```python
from build123d import *

# Parameters (mm, degrees)
SKETCH2_W           = 15
SKETCH2_H           = 15
BOSS_EXTRUDE1_DEPTH = 15
FILLET1_R           = 6.35


with BuildPart() as part:
    # Sketch2 → Boss-Extrude1 (new body)
    with BuildSketch(Plane.XY):
        Polygon((75, 0), (75, -200), (25, -200), (25, 0), (25, 18.884295249), (0, 62.185565438), (25, 62.185565438), (25, 64.822440103), (0, 108.123710292), (25, 108.123710292), (25, 110.760584957), (0, 154.061855146), (25, 154.061855146), (25, 156.698729811), (0, 200), (100, 200), (75, 156.698729811), (75, 154.061855146), (100, 154.061855146), (75, 110.760584957), (75, 108.123710292), (100, 108.123710292), (75, 64.822440103), (75, 62.185565438), (100, 62.185565438), (75, 18.884295249), align=None)
        with Locations((50, -170)):
            Rectangle(SKETCH2_W, SKETCH2_H, mode=Mode.SUBTRACT)
        with Locations((50, -30)):
            Rectangle(SKETCH2_W, SKETCH2_H, mode=Mode.SUBTRACT)
        with Locations((50, 175)):
            Rectangle(SKETCH2_W, SKETCH2_H, mode=Mode.SUBTRACT)
    extrude(amount=-BOSS_EXTRUDE1_DEPTH)

    # Fillet1
    fillet1_edges = [part.edges().sort_by_distance(p)[0] for p in [
        (0, 62.185565438, -7.5),
        (0, 108.123710292, -7.5),
        (0, 154.061855146, -7.5),
        (0, 200, -7.5),
        (100, 200, -7.5),
        (100, 154.061855146, -7.5),
        (100, 108.123710292, -7.5),
        (100, 62.185565438, -7.5),
    ]]
    fillet(fillet1_edges, radius=FILLET1_R)


solid = part.part
```
Here's how the part is built. I have some questions about the finished solid (model axes, mm). A direction names the side the tool comes from. Coordinates: 2 decimals unless noted, no trailing zeros. Order: outer loops, then holes, each group sorted by start corner. A loop starts at its lowest first (then second) coordinate and runs counter-clockwise, first axis right, second up.
Item 1: Thinking about a two-plate mould opening in X: for faces 1 (the face through (50, 182.5, -7)), 2 (the face through (5.453, 58.93, -7.605)), 3 (the face through (94.547, 150.806, -7.605)), which applies, pulls with the +X half, pulls with the -X half, needs draft (parallel to the pull), parting line crosses it, or undercut?
Response values:
face 1: undercut
face 2: pulls with the -X half
face 3: pulls with the +X half
Item 2: Which directions (+Z, -Z, +X, -X, +Y, -Y) give clear straight access to the entire face, cutting with the end or side of a thin tool? Please do faces 4 (the face through (15.386, 127.412, -7.395)), 5 (the face through (75, -92, -7)), 6 (the face through (82, 154.062, -7)), 7 (the face through (50, -177.5, -7)), 8 (the face through (51, 3, 0)).
Response values:
face 4: +Z, -Z, -X
face 5: +Z, -Z, +X, -Y
face 6: +Z, -Z, +X
face 7: +Z, -Z
face 8: +Z, +X, -X, +Y, -Y
Item 3: If we section it at C-C, the plane y = -96: List the corners of the cut face in (x, z) for me, then the cut area to 3 significant figures.
Response values:
outline: (25, -15) - (75, -15) - (75, 0) - (25, 0) - close
area: 750 mm2
Item 4: If we section it at A-A, the plane x = 18.5: List the corners of the cut face in (y, z) for me, then the cut area to 3 significant figures.
Response values:
outline: (30.14, -15) - (62.19, -15) - (62.19, 0) - (30.14, 0) - close; (76.08, -15) - (108.12, -15) - (108.12, 0) - (76.08, 0) - close; (122.02, -15) - (154.06, -15) - (154.06, 0) - (122.02, 0) - close; (167.96, -15) - (200, -15) - (200, 0) - (167.96, 0) - close
area: 1,920 mm2
Item 5: If we section it at D-D, the plane y = 124.5: List the corners of the cut face in (x, z) for me, then the cut area to 3 significant figures.
Response values:
outline: (17.07, -15) - (82.93, -15) - (82.93, 0) - (17.07, 0) - close
area: 988 mm2
Item 6: I need wall thicknesses on probe 1 along Y at (x, z) = (56.5, -7); probe 2 along Y at (x, z) = (22.5, -10.75); probe 3 along X at (y, z) = (-164.5, -10.5). Which ranges of each line are inside material? Lowest first, please.
Response values:
probe 1: y = -200 to -177.5, -162.5 to -37.5, -22.5 to 167.5, 182.5 to 200
probe 2: y = 23.21 to 62.19, 69.15 to 108.12, 115.09 to 154.06, 161.03 to 200
probe 3: x = 25 to 42.5, 57.5 to 75
Item 7: I'm going to push flat-ended pins straight in: pin 1 Ø2 at (y, z) = (-29.5, -1.5) entering from -X; pin 2 Ø7.5 at (y, z) = (177.5, -11) entering from +X; pin 3 Ø0.8 at (y, z) = (63, -9) entering from +X. Where does each tip first touch, or does it pass through?
Response values:
pin 1: stops at x = 25
pin 2: stops at x = 89.17
pin 3: stops at x = 75
Item 8: If we section it at B-B, the plane z = -7.5: Give the number of separate pieces and of enclosed holes in the cut face, then the cut area to 3 significant figures.
Response values:
separate pieces: 1
enclosed holes: 3
area: 23,400 mm2
